The listing builds one solid part. Answer for the finished solid, in the listing's coordinates (mm). A direction names the side the tool comes from. Coordinates: 2 decimals unless noted, no trailing zeros. Loops run counter-clockwise (first coordinate to the right, second up) from the corner with the lowest first, then second, coordinate; pieces in that order, holes last. Notation, with made-up numbers: (46, 17.25) - (90, 17.25) arc R3 cw to (90, 21.25) - close; hole circle Ø9 at (22, -31.75). An arc over 180 degrees is marked (long way). Return JSON: item names as keys, results as strings. Group by question number.
1. Find the intervals of material crossed by line 1 along Z through (x, y) = (6.35, -0.5); line 2 along X through (y, z) = (3, 4) (3 decimals); line 3 along Y through (x, z) = (0, 3) (1 decimal), in increasing order.
2. Section B-B (z = 3.5) is taken. Write down the section's boundary in (x, y) (1 decimal), and give its area (3 significant figures).
3. Each of these flat-tipped pins is pushed along its axis until it touches: P1, Ø1.9, axis at x = -7, z = 2, coming from the +Y side (3 decimals); P2, Ø1, axis at y = 5, z = 2, coming from the -X side (3 decimals). Where does it stop, or does it pass through?
4. Which of the six approach directions +Z, -Z, +X, -X, +Y, -Y give full straight-line access (tool end or side, diameter ignored) to faces 4 (the face through (3.175, 6, 3)), 5 (the face through (-3.175, 6, 3)), 6 (the face through (0, -3.175, 3))?
5. Section C-C (y = 0.25) is taken. Write down the section's boundary in (x, z) (3 decimals), and give its area (3 significant figures).
6. Section D-D (x = 6.35) is taken. Write down the section's boundary in (y, z) (3 decimals).
7. The mould has two halves that part along X. Classify faces 1 (the face through (9.525, 0, 3)), 2 (the face through (0, 7.938, 3)), 3 (the face through (0.192, 6.223, 3.131)): pulls with the +X half, pulls with the -X half, needs draft (parallel to the pull), parting line crosses it, or undercut.
```python
from build123d import *

# Parameters (mm, degrees)
SKETCH1_W                        = 19.05
SKETCH1_H                        = 6.35
BOSS_EXTRUDE1_DEPTH              = 6.35
SKETCH6_W                        = 6.35
SKETCH6_H                        = 6.35
BOSS_EXTRUDE2_DEPTH              = 4.7625
TAPPED_HOLE_FOR_4_40_HELICOIL1_D = 3.048
F_4_CLEARANCE_HOLE2_D            = 2.9464


with BuildPart() as part:
    # Sketch1 → Boss-Extrude1 (new body)
    with BuildSketch(Plane.XY):
        Rectangle(SKETCH1_W, SKETCH1_H)
    extrude(amount=BOSS_EXTRUDE1_DEPTH)

    # Sketch6 → Boss-Extrude2 (add)
    with BuildSketch(Plane(origin=(0, 3.175, 0), x_dir=(1, 0, 0), z_dir=(0, 1, 0))):
        with Locations((0, -3.175)):
            Rectangle(SKETCH6_W, SKETCH6_H)
    extrude(amount=BOSS_EXTRUDE2_DEPTH)

    # Tapped Hole for #4-40 Helicoil1 (through all)
    with Locations(Plane(origin=(0, 3.175, 0), x_dir=(1, 0, 0), z_dir=(0, 1, 0))):
        with Locations((-6.35, -3.175), (6.35, -3.175)):
            Hole(TAPPED_HOLE_FOR_4_40_HELICOIL1_D / 2)

    # #4 Clearance Hole2 (through all)
    with Locations(Plane.XY.offset(6.35)):
        with Locations((0, 4.7625)):
            Hole(F_4_CLEARANCE_HOLE2_D / 2)


solid = part.part
```
The answers:
{
 "1": {"line 1": "z = 0 to 1.65, 4.7 to 6.35", "line 2": "x = -9.525 to -7.631, -5.069 to 5.069, 7.631 to 9.525", "line 3": "y = -3.2 to 3.3, 6.2 to 7.9"},
 "2": {"outline": "(-9.5, -3.2) - (-7.8, -3.2) - (-7.8, 3.2) - (-9.5, 3.2) - close; (-4.9, -3.2) - (4.9, -3.2) - (4.9, 3.2) - (3.2, 3.2) - (3.2, 7.9) - (-3.2, 7.9) - (-3.2, 3.2) - (-4.9, 3.2) - close; (7.8, -3.2) - (9.5, -3.2) - (9.5, 3.2) - (7.8, 3.2) - close; hole circle Ø2.9 at (0, 4.8)", "area": "107 mm2"},
 "3": {"P1": "stops at y = 3.175", "P2": "stops at x = -3.175"},
 "4": {"face 4": "+Z, -Z, +X, +Y", "face 5": "+Z, -Z, -X, +Y", "face 6": "+Z, -Z, +X, -X, -Y"},
 "5": {"outline": "(-9.525, 0) - (9.525, 0) - (9.525, 6.35) - (-9.525, 6.35) - close; hole circle Ø3.048 at (-6.35, 3.175); hole circle Ø3.048 at (6.35, 3.175)", "area": "106 mm2"},
 "6": {"outline": "(-3.175, 0) - (3.175, 0) - (3.175, 1.651) - (-3.175, 1.651) - close; (-3.175, 4.699) - (3.175, 4.699) - (3.175, 6.35) - (-3.175, 6.35) - close"},
 "7": {"face 1": "pulls with the +X half", "face 2": "needs draft", "face 3": "undercut"}
}
